The listing builds one solid part. Answer for the finished solid, in the listing's coordinates (mm). Face numbers are marked on the shaded views. A direction names the side the tool comes from. Give positions to 0.01 mm unless a question says otherwise; leave off trailing zeros. Order: outer loops, then holes, each group sorted by start corner. A loop starts at its lowest first (then second) coordinate and runs counter-clockwise, first axis right, second up. Notation, with made-up numbers: (77, 88) - (135, 88) arc R33 ccw to (135, 127) - close; hole circle Ø2 at (-31.5, 30.5). An arc over 180 degrees is marked (long way). Use a Markdown table: item, result. Add a question column.
1) The mould has two halves that part along Z. Classify the marked faces 1, 2 and 3: released by +Z, released by -Z, zero draft, split by the parting line, or undercut.
2) Find section B-B, the plane z = 0. Determine the outline of the cut face in (x, y), plus the area to 3 significant figures.
3) Find section C-C, the plane y = 28.5. Determine the outline of the cut face in (x, z).
4) Find section D-D, the plane z = -14. Determine the outline of the cut face in (x, y).
5) Flat-ended cylindrical pins translate along their axes: pin 1 (7 mm diameter, centred on y = 27, z = -13.5, fed in from +X); pin 2 (20 mm diameter, centred on x = -68, z = 8.5, fed in from +Y). Find the tip coordinate at first contact, or state that the pin passes through.
6) Find section A-A, the plane y = 14.5. Determine the outline of the cut face in (x, z).
7) Straight lines are drawn through the part: line 1 (Z direction, x = -65, y = 23.5); line 2 (Y direction, x = -25, z = -15.5); line 3 (Z direction, x = -19, y = 2). For each, find the intervals that lie inside material, in ascending order.
8) For the marked faces 4, 5 and 6, determine the directions among +Z, -Z, +X, -X, +Y, -Y from which every point of the face is accessible in a straight line to the end or side of a thin tool.
from build123d import *

# Parameters (mm, degrees)
BOSS_EXTRUDE1_DEPTH = 9
SKETCH2_3_W         = 35
SKETCH2_3_H         = 9
BOSS_EXTRUDE2_DEPTH = 55.5
CUT_EXTRUDE1_DEPTH  = 55.5


with BuildPart() as part:
    # Sketch2 → Boss-Extrude1 (new body)
    with BuildSketch(Plane(origin=(0, 0, 0), x_dir=(1, 0, 0), z_dir=(0, 1, 0))):
        with BuildLine():
            Line((-12.051133951, 20), (-63.051133951, 20))
            Line((-63.051133951, 20), (-63.051133951, 11))
            Line((-63.051133951, 11), (-98.051133951, 11))
            Line((-98.051133951, 11), (-98.051133951, -11))
            Line((-98.051133951, -11), (-63.051133951, -11))
            Line((-63.051133951, -11), (-63.051133951, -20))
            Line((-63.051133951, -20), (-12.051133951, -20))
            ThreePointArc((-12.051133951, -20), (7.948866049, 0), (-12.051133951, 20))
        make_face()
        with BuildLine():
            ThreePointArc((-12.051133951, 7), (-5.051133951, 0), (-12.051133951, -7))
            Line((-12.051133951, -7), (-35.051133951, -7))
            ThreePointArc((-35.051133951, -7), (-42.051133951, 0), (-35.051133951, 7))
            Line((-35.051133951, 7), (-12.051133951, 7))
        make_face(mode=Mode.SUBTRACT)
    extrude(amount=BOSS_EXTRUDE1_DEPTH)

    # Sketch2_3 → Boss-Extrude2 (add)
    with BuildSketch(Plane(origin=(0, 0, 0), x_dir=(1, 0, 0), z_dir=(0, 1, 0))):
        with Locations((-80.551133951, -15.5)):
            Rectangle(SKETCH2_3_W, SKETCH2_3_H)
        with Locations((-80.551133951, 15.5)):
            Rectangle(SKETCH2_3_W, SKETCH2_3_H)
    extrude(amount=BOSS_EXTRUDE2_DEPTH)

    # Sketch3 → Cut-Extrude1 (cut)
    with BuildSketch(Plane.XY.offset(20)):
        with BuildLine():
            ThreePointArc((-98.051133951, 33.947689481), (-80.551133951, 51.447689481), (-63.051133951, 33.947689481))
            Line((-63.051133951, 33.947689481), (-63.051133951, 55.5))
            Line((-63.051133951, 55.5), (-98.051133951, 55.5))
            Line((-98.051133951, 55.5), (-98.051133951, 33.947689481))
        make_face()
        with BuildLine():
            ThreePointArc((-87.551133951, 33.947689481), (-80.551133951, 26.947689481), (-73.551133951, 33.947689481))
            Line((-73.551133951, 33.947689481), (-87.551133951, 33.947689481))
        make_face()
        with BuildLine():
            Line((-87.551133951, 33.947689481), (-73.551133951, 33.947689481))
            ThreePointArc((-73.551133951, 33.947689481), (-80.551133951, 40.947689481), (-87.551133951, 33.947689481))
        make_face()
    extrude(amount=-CUT_EXTRUDE1_DEPTH, mode=Mode.SUBTRACT)


solid = part.part
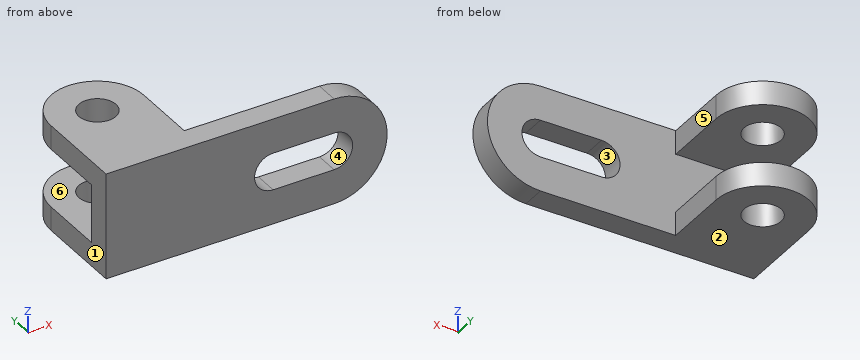
The answers:
| question | item | result |
|---|---|---|
| 1 | face 1 | zero draft |
| 1 | face 2 | released by -Z |
| 1 | face 3 | undercut |
| 2 | outline | (-98.05, 0) - (-42.05, 0) - (-42.05, 9) - (-98.05, 9) - close; (-5.05, 0) - (7.95, 0) - (7.95, 9) - (-5.05, 9) - close |
| 2 | area | 621 mm2 |
| 3 | outline | (-98.05, -20) - (-84.95, -20) - (-84.95, -11) - (-98.05, -11) - close; (-98.05, 11) - (-84.95, 11) - (-84.95, 20) - (-98.05, 20) - close; (-76.16, -20) - (-63.05, -20) - (-63.05, -11) - (-76.16, -11) - close; (-76.16, 11) - (-63.05, 11) - (-63.05, 20) - (-76.16, 20) - close |
| 4 | outline | (-98.05, 0) - (2.23, 0) - (2.23, 9) - (-63.05, 9) - (-63.05, 33.95) arc R17.5 ccw to (-98.05, 33.95) - close; hole circle Ø14 at (-80.55, 33.95) |
| 5 | pin 1 | x = -63.05 |
| 5 | pin 2 | y = 51.21 |
| 6 | outline | (-98.05, -20) - (-63.05, -20) - (-63.05, -11) - (-98.05, -11) - close; (-98.05, 11) - (-63.05, 11) - (-63.05, 20) - (-98.05, 20) - close |
| 7 | line 1 | -20 to -11, 11 to 20 |
| 7 | line 2 | 0 to 9 |
| 7 | line 3 | -20 to -7, 7 to 20 |
| 8 | face 4 | +Y, -Y |
| 8 | face 5 | +Z, -Z, +X, +Y |
| 8 | face 6 | +X, -X, +Y |
